Check sheet for the modelled part. Datum: model origin and axes. Units: mm. A direction names the side the tool comes from. Coordinates: 2 decimals unless noted, no trailing zeros. Use a Markdown table: item, result. Add a question column.
1) Thickness scan on line 1 (Y direction, x = 75, z = 3); line 2 (Y direction, x = -7.5, z = 5.75) (3 decimals); line 3 (X direction, y = 17, z = 4). Record the ranges inside material, lowest first.
2) Sectioned sample at A-A, the plane z = 3.25. State how many separate pieces and enclosed holes the cut face has, then the cut area to 3 significant figures.
3) Tool access check on faces 1 (the flat face through (30, -16.825, 3)), 2 (the flat face through (-2, 1, 6.35)). Record the directions out of +Z, -Z, +X, -X, +Y, -Y that give a thin tool (end or side, any length) a straight path to the whole face; none if there is none.
4) Draft check along Y on faces 3 (the cylindrical face through (143.769, 72.594, 3.131)), 4 (the cylindrical face through (73.1, -18.3, 3.1)), 5 (the flat face through (-2, 1, 0)). Enter one of: pulls with the +Y half, pulls with the -Y half, needs draft (parallel to the pull), parting line crosses it, or undercut.
from build123d import *

# Parameters (mm, degrees)
F0_R     = 2.55
F0_W     = 50
F0_H     = 6.35
F1_DEPTH = 6.35


with BuildPart() as f1:
    # F0 (on Top) → F1 (new body)
    with BuildSketch(Plane.XY):
        with BuildLine():
            ThreePointArc((146.05, 67), (143.706854, 72.656854), (138.05, 75))
            Line((138.05, 75), (-138.05, 75))
            ThreePointArc((-138.05, 75), (-143.706854, 72.656854), (-146.05, 67))
            Line((-146.05, 67), (-146.05, -67))
            ThreePointArc((-146.05, -67), (-143.706854, -72.656854), (-138.05, -75))
            Line((-138.05, -75), (138.05, -75))
            ThreePointArc((138.05, -75), (143.706854, -72.656854), (146.05, -67))
            Line((146.05, -67), (146.05, 67))
        make_face()
        with Locations((-75, -20)):
            Circle(F0_R, mode=Mode.SUBTRACT)
        with Locations((-30, -20)):
            Rectangle(F0_W, F0_H, mode=Mode.SUBTRACT)
        with Locations((30, -20)):
            Rectangle(F0_W, F0_H, mode=Mode.SUBTRACT)
        with Locations((75, -20)):
            Circle(F0_R, mode=Mode.SUBTRACT)
        with Locations((-75, 20)):
            Circle(F0_R, mode=Mode.SUBTRACT)
        with Locations((-30, 20)):
            Rectangle(F0_W, F0_H, mode=Mode.SUBTRACT)
        with Locations((30, 20)):
            Rectangle(F0_W, F0_H, mode=Mode.SUBTRACT)
        with Locations((75, 20)):
            Circle(F0_R, mode=Mode.SUBTRACT)
    extrude(amount=F1_DEPTH)


solid = f1.part
Solved:
| question | item | result |
|---|---|---|
| 1 | line 1 | y = -75 to -22.55, -17.45 to 17.45, 22.55 to 75 |
| 1 | line 2 | y = -75 to -23.175, -16.825 to 16.825, 23.175 to 75 |
| 1 | line 3 | x = -146.05 to -55, -5 to 5, 55 to 146.05 |
| 2 | separate pieces | 1 |
| 2 | enclosed holes | 8 |
| 2 | area | 42,400 mm2 |
| 3 | face 1 | +Z, -Z |
| 3 | face 2 | +Z, +X, -X, +Y, -Y |
| 4 | face 3 | pulls with the +Y half |
| 4 | face 4 | undercut |
| 4 | face 5 | needs draft |
